```python
from build123d import *

# Parameters (mm, degrees)
SKETCH1_W                   = 35
SKETCH1_H                   = 12.06
BOSS_EXTRUDE1_DEPTH         = 5
M5_CLEARANCE_HOLE1_D        = 5.8
TAP_DRILL_FOR_M3X0_5_TAP1_D = 2.5
SKETCH7_W                   = 35
SKETCH7_H                   = 8
BOSS_EXTRUDE2_DEPTH         = 2


with BuildPart() as part:
    # Sketch1 → Boss-Extrude1 (new body)
    with BuildSketch(Plane(origin=(0, 0, 0), x_dir=(1, 0, 0), z_dir=(0, 1, 0))):
        Rectangle(SKETCH1_W, SKETCH1_H)
    extrude(amount=BOSS_EXTRUDE1_DEPTH)

    # M5 Clearance Hole1 (through all)
    with Locations(Plane(origin=(0, 5, 0), x_dir=(1, 0, 0), z_dir=(0, 1, 0))):
        with Locations((13.5, 0)):
            Hole(M5_CLEARANCE_HOLE1_D / 2)

    # Tap Drill for M3x0.5 Tap1 (through all)
    with Locations(Plane(origin=(0, 5, 0), x_dir=(1, 0, 0), z_dir=(0, 1, 0))):
        with Locations((-1.9, 0), (-11.9, 0)):
            Hole(TAP_DRILL_FOR_M3X0_5_TAP1_D / 2)

    # Sketch7 → Boss-Extrude2 (add)
    with BuildSketch(Plane(origin=(0, 0, -6.03), x_dir=(-1, 0, 0), z_dir=(0, 0, -1))):
        with Locations((0, 1)):
            Rectangle(SKETCH7_W, SKETCH7_H)
    extrude(amount=BOSS_EXTRUDE2_DEPTH)

    # Mirror1: part across plane


with BuildPart() as part_1:
    add(part.part)
    add(part.part.mirror(Plane.XY))


solid = part_1.part
```
Model file for the job. Use its own axes, mm. A direction names the side the tool comes from. Give positions to 0.01 mm unless a question says otherwise; leave off trailing zeros. Order: outer loops, then holes, each group sorted by start corner. A loop starts at its lowest first (then second) coordinate and runs counter-clockwise, first axis right, second up.
1) Wall check: probe 1 along X at (y, z) = (3, 0); probe 2 along Z at (x, y) = (-11.9, 1.95); probe 3 along Z at (x, y) = (5, -1.5). Give the ranges that are in metal, low to high.
2) Saw through at D-D, the plane y = -2. Write the cut outline in (x, z), then the cut area to 3 significant figures.
3) Mould opens along X. For faces 1 (the flat face through (0, 1, -8.03)), 2 (the flat face through (-17.5, 2, 0)), 3 (the cylindrical face through (-0.65, 2.47, -0.05)) say: +X half, -X half, draft (parallel to the pull), parting line (faces both ways), or undercut.
4) Pin check, flat tip, straight feed: pin 1 (3 mm diameter, centred on x = -1.9, z = 0, fed in from +Y). Stop position of the tip, or through.
5) Saw through at B-B, the plane z = 0. Write the cut outline in (x, y).
6) Saw through at C-C, the plane x = 13.5. Write the cut outline in (y, z), then the cut area to 3 significant figures.
7) 3-axis set-ups, long thin cutter, end or side, ignore diameter. For faces 4 (the cylindrical face through (16.4, 2.5, -0.1)), 5 (the flat face through (0, -1, 6.03)): which of +Z, -Z, +X, -X, +Y, -Y reach the whole face in a straight line?
8) Saw through at A-A, the plane y = 3.25. Write the cut outline in (x, z), then the cut area to 3 significant figures.
Computed:
1. probe 1: x = -17.5 to -13.15, -10.65 to -3.15, -0.65 to 10.6, 16.4 to 17.5
1. probe 2: z = -8.03 to -1.25, 1.25 to 8.03
1. probe 3: z = -8.03 to -6.03, 6.03 to 8.03
2. outline: (-17.5, -8.03) - (17.5, -8.03) - (17.5, -6.03) - (-17.5, -6.03) - close; (-17.5, 6.03) - (17.5, 6.03) - (17.5, 8.03) - (-17.5, 8.03) - close
2. area: 140 mm2
3. face 1: draft
3. face 2: -X half
3. face 3: undercut
4. pin 1: stops at y = 5
5. outline: (-17.5, 0) - (-13.15, 0) - (-13.15, 5) - (-17.5, 5) - close; (-10.65, 0) - (-3.15, 0) - (-3.15, 5) - (-10.65, 5) - close; (-0.65, 0) - (10.6, 0) - (10.6, 5) - (-0.65, 5) - close; (16.4, 0) - (17.5, 0) - (17.5, 5) - (16.4, 5) - close
6. outline: (-3, -8.03) - (5, -8.03) - (5, -2.9) - (0, -2.9) - (0, -6.03) - (-3, -6.03) - close; (-3, 6.03) - (0, 6.03) - (0, 2.9) - (5, 2.9) - (5, 8.03) - (-3, 8.03) - close
6. area: 63.3 mm2
7. face 4: +Y, -Y
7. face 5: +X, -X, -Y
8. outline: (-17.5, -8.03) - (17.5, -8.03) - (17.5, 8.03) - (-17.5, 8.03) - close; hole circle Ø2.5 at (-11.9, 0); hole circle Ø2.5 at (-1.9, 0); hole circle Ø5.8 at (13.5, 0)
8. area: 526 mm2
